Could you check a few things on this model? Use its own coordinates, in mm. Coordinates: 2 decimals unless noted, no trailing zeros. Loops run counter-clockwise (first coordinate to the right, second up) from the corner with the lowest first, then second, coordinate; pieces in that order, holes last.
1) Will this pin go through, and if not, where does the flat tip stop? P1, Ø4, axis at x = 13.5, z = 15.5, coming from the +Y side.
2) If I drill on line 1 along X through (y, z) = (4.75, 15); line 2 along Y through (x, z) = (14.5, -13), over which ranges is the centre line in solid material (lowest first)?
3) Imagine slicing it at B-B on z = -15. Please give me the cut outline in (x, y), plus the area to 3 significant figures.
4) Imagine slicing it at C-C on y = 11.75. Please give me the cut outline in (x, z).
5) Imagine slicing it at A-A on x = -15. Please give me the cut outline in (y, z).
```python
from build123d import *

# Parameters (mm, degrees)
SKETCH1_W                             = 50
SKETCH1_H                             = 50
BOSS_EXTRUDE1_DEPTH                   = 15
TAP_DRILL_FOR_M4X0_7_TAP1_D           = 3.3
TAP_DRILL_FOR_M4X0_7_TAP1_CSINK_D     = 3.35
TAP_DRILL_FOR_M4X0_7_TAP1_CSINK_ANGLE = 90
SKETCH3_W                             = 8
SKETCH3_H                             = 8
CUT_EXTRUDE2_DEPTH                    = 5


with BuildPart() as part:
    # Sketch1 → Boss-Extrude1 (new body)
    with BuildSketch(Plane(origin=(0, 0, 0), x_dir=(1, 0, 0), z_dir=(0, 1, 0))):
        Rectangle(SKETCH1_W, SKETCH1_H)
    extrude(amount=BOSS_EXTRUDE1_DEPTH)

    # Tap Drill for M4x0.7 Tap1 (through all)
    with Locations(Plane(origin=(0, 15, 0), x_dir=(1, 0, 0), z_dir=(0, 1, 0))):
        with Locations((-15, 15), (15, 15), (15, -15), (-15, -15)):
            CounterSinkHole(TAP_DRILL_FOR_M4X0_7_TAP1_D / 2, TAP_DRILL_FOR_M4X0_7_TAP1_CSINK_D / 2, counter_sink_angle=TAP_DRILL_FOR_M4X0_7_TAP1_CSINK_ANGLE)

    # Sketch3 → Cut-Extrude2 (cut)
    with BuildSketch(Plane(origin=(0, 15, 0), x_dir=(1, 0, 0), z_dir=(0, 1, 0))):
        with Locations((15, 15)):
            Rectangle(SKETCH3_W, SKETCH3_H)
        with Locations((-15, 15)):
            Rectangle(SKETCH3_W, SKETCH3_H)
        with Locations((-15, -15)):
            Rectangle(SKETCH3_W, SKETCH3_H)
        with Locations((15, -15)):
            Rectangle(SKETCH3_W, SKETCH3_H)
    extrude(amount=-CUT_EXTRUDE2_DEPTH, mode=Mode.SUBTRACT)


solid = part.part
```
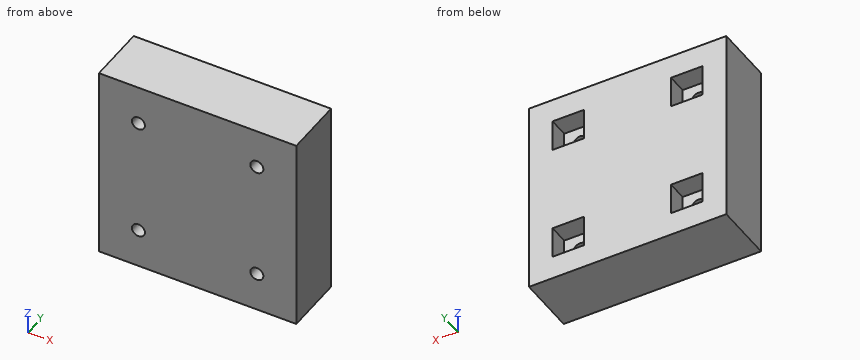
Filled in:
1. P1: stops at y = 10
2. line 1: x = -25 to -16.65, -13.35 to 13.35, 16.65 to 25
2. line 2: y = 0 to 10
3. outline: (-25, 0) - (-16.65, 0) - (-16.65, 10) - (-19, 10) - (-19, 15) - (-25, 15) - close; (-13.35, 0) - (13.35, 0) - (13.35, 10) - (11, 10) - (11, 15) - (-11, 15) - (-11, 10) - (-13.35, 10) - close; (16.65, 0) - (25, 0) - (25, 15) - (19, 15) - (19, 10) - (16.65, 10) - close
3. area: 604 mm2
4. outline: (-25, -25) - (25, -25) - (25, 25) - (-25, 25) - close; hole (-19, -19) - (-11, -19) - (-11, -11) - (-19, -11) - close; hole (-19, 11) - (-11, 11) - (-11, 19) - (-19, 19) - close; hole (11, -19) - (19, -19) - (19, -11) - (11, -11) - close; hole (11, 11) - (19, 11) - (19, 19) - (11, 19) - close
5. outline: (0, -25) - (15, -25) - (15, -19) - (10, -19) - (10, -16.65) - (0, -16.65) - close; (0, -13.35) - (10, -13.35) - (10, -11) - (15, -11) - (15, 11) - (10, 11) - (10, 13.35) - (0, 13.35) - close; (0, 16.65) - (10, 16.65) - (10, 19) - (15, 19) - (15, 25) - (0, 25) - close
